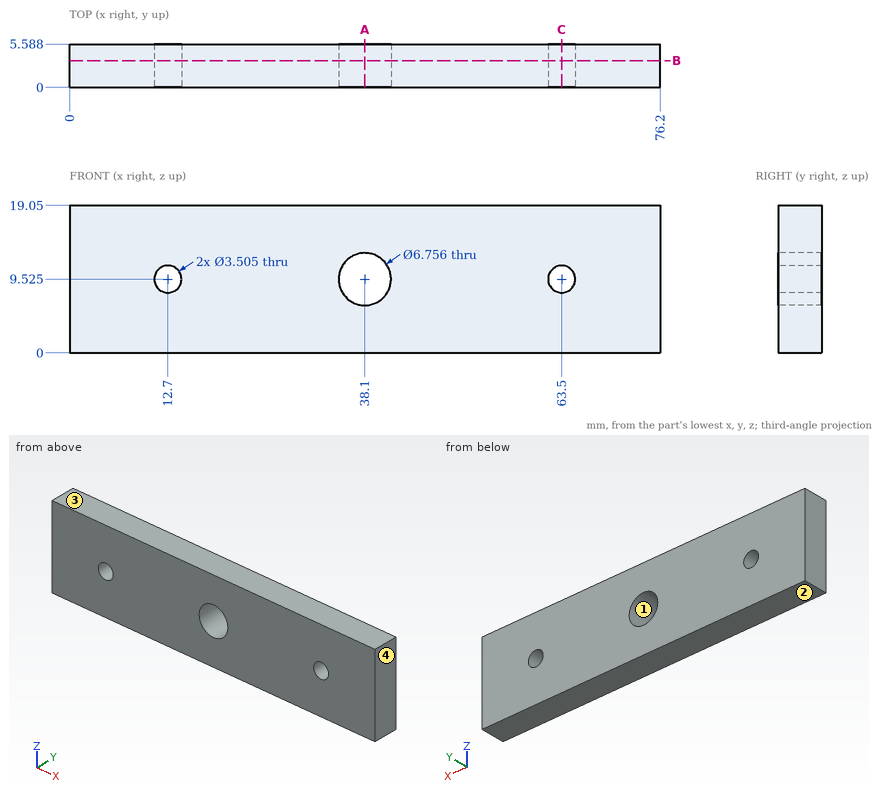
Answer from the drawing. Dimensions are ordinates in mm from the lowest x, y and z of the part. Round coordinates to 2 decimals unless told otherwise and drop trailing zeros. Write each loop counter-clockwise with the first axis right and the second up, starting at its lowest first coordinate (ties: lowest second). Pieces come first, ordered by that corner, then holes. Notation, with made-up numbers: M 26,-26.5 L 47,-26.5 A24 ccw 47,-16.5 Z; hole C 8,20 d5. An arc over 180 degrees is marked long. One line per item, written item: value.
Q1. Find section C-C on x = 63.5. Write down the section's boundary in (y, z).
Data:
outline: M 0,0 L 5.59,0 L 5.59,7.77 L 0,7.77 Z; M 0,11.28 L 5.59,11.28 L 5.59,19.05 L 0,19.05 Z
Q2. Straight lines are drawn through the part: line 1 (Z direction, x = 63.5, y = 3.65); line 2 (Z direction, x = 38.1, y = 3.7); line 3 (X direction, y = 2.8, z = 8) (1 decimal). For each, find the intervals that lie inside material, in ascending order. Write a range as [from, to].
Data:
line 1: [0, 7.77], [11.28, 19.05]
line 2: [0, 6.15], [12.9, 19.05]
line 3: [0, 11.8], [13.6, 35.1], [41.1, 62.6], [64.4, 76.2]
Q3. Find section B-B on y = 3.45. Count the separate pieces of the cut face and the enclosed holes in it, plus the area to 3 significant figures.
Data:
separate pieces: 1
enclosed holes: 3
area: 1,400 mm2
Q4. For a pull along Z with two mould halves and no side action, classify the marked faces 1, 2, 3 and 4 as +Z half, -Z half, draft (parallel to the pull), parting line (faces both ways), or undercut.
Data:
face 1: undercut
face 2: -Z half
face 3: +Z half
face 4: draft
Q5. Find section A-A on x = 38.1. Write down the section's boundary in (y, z).
Data:
outline: M 0,0 L 5.59,0 L 5.59,6.15 L 0,6.15 Z; M 0,12.9 L 5.59,12.9 L 5.59,19.05 L 0,19.05 Z
